Part model, mm, in its own coordinate system. Give positions to 0.01 mm unless a question says otherwise; leave off trailing zeros. Order: outer loops, then holes, each group sorted by start corner. A loop starts at its lowest first (then second) coordinate and runs counter-clockwise, first axis right, second up. Notation, with made-up numbers: (74, -11) - (87, -11) arc R10 cw to (87, -4) - close; hole circle Ø8 at (-17.5, -27). An arc over 180 degrees is marked (long way). One line per item, written item: value.
```python
from build123d import *

# Parameters (mm, degrees)
BOSS_EXTRUDE1_DEPTH     = 28.2702
SKETCH2_R               = 3.556
SKETCH2_R_2             = 1.4986
SKETCH2_R_3             = 2.0066
MOTOR_MOUNT_HOLES_DEPTH = 50.437835996
SKETCH3_R               = 1.7018
PLATE_MOUNT_HOLES_DEPTH = 51.700550556
SKETCH4_W               = 28.2702
SKETCH4_H               = 29.2608
CUT_EXTRUDE1_DEPTH      = 50.437835996
FILLET1_R               = 1.905


with BuildPart() as part:
    # Sketch1 → Boss-Extrude1 (new body)
    with BuildSketch(Plane(origin=(0, 0, 0), x_dir=(0, 0, -1), z_dir=(1, 0, 0))):
        Polygon((0, 0), (0, -30.1498), (-30.2514, -30.1498), (-30.2514, -29.2608), (-3.1242, -29.2608), (-3.1242, 0), align=None)
    extrude(amount=BOSS_EXTRUDE1_DEPTH)

    # Sketch2 → Motor_Mount_holes (cut, through all)
    with BuildSketch(Plane.XY.offset(3.1242)):
        with Locations((14.1351, -11.6586)):
            Circle(SKETCH2_R)
        with Locations((14.1351, -3.1496)):
            Circle(SKETCH2_R_2)
        with Locations((5.2451, -11.6586)):
            Circle(SKETCH2_R_3)
        with Locations(Location((23.0251, -11.6586, 0), (0, 0, 180))):
            Circle(SKETCH2_R_3)
        with Locations(Location((14.1351, -20.1676, 0), (0, 0, 180))):
            Circle(SKETCH2_R_2)
    extrude(amount=-MOTOR_MOUNT_HOLES_DEPTH, mode=Mode.SUBTRACT)

    # Sketch3 → Plate_Mount_Holes (cut, through all)
    with BuildSketch(Plane(origin=(0, -29.2608, 0), x_dir=(1, 0, 0), z_dir=(0, 1, 0))):
        with Locations(Location((24.3205, -7.7597, 0), (0, 0, 270))):
            Circle(SKETCH3_R)
        with Locations(Location((3.9497, -7.7597, 0), (0, 0, 90))):
            Circle(SKETCH3_R)
        with Locations(Location((3.9497, -21.3741, 0), (0, 0, 270))):
            Circle(SKETCH3_R)
        with Locations(Location((24.3205, -21.3741, 0), (0, 0, 90))):
            Circle(SKETCH3_R)
    extrude(amount=-PLATE_MOUNT_HOLES_DEPTH, mode=Mode.SUBTRACT)

    # Sketch4 → Cut-Extrude1 (cut, through all)
    with BuildSketch(Plane.XY.offset(3.1242)):
        with Locations((14.1351, -14.6304)):
            Rectangle(SKETCH4_W, SKETCH4_H)
    extrude(amount=-CUT_EXTRUDE1_DEPTH, mode=Mode.SUBTRACT)

    # Fillet1
    fillet1_edges = [part.edges().sort_by_distance(p)[0] for p in [
        (28.2702, -29.7053, 30.2514),
        (28.2702, -29.7053, 0),
        (0, -29.7053, 0),
        (0, -29.7053, 30.2514),
    ]]
    fillet(fillet1_edges, radius=FILLET1_R)


solid = part.part
```
1) Pin check, flat tip, straight feed: pin 1 (3 mm diameter, centred on x = 3.95, z = 7.76, fed in from -Y). Stop position of the tip, or through.
Outcome:
pin 1: passes through
2) Cut at A-A, the plane x = 25. Give the cut face in (y, z).
Outcome:
outline: (-30.15, 0) - (-29.26, 0) - (-29.26, 6.2) - (-30.15, 6.2) - close; (-30.15, 9.32) - (-29.26, 9.32) - (-29.26, 19.81) - (-30.15, 19.81) - close; (-30.15, 22.93) - (-29.26, 22.93) - (-29.26, 30.25) - (-30.15, 30.25) - close
3) Mould opens along Z. For faces 1 (the cylindrical face through (0.573, -29.712, 0.543)), 2 (the flat face through (14, -30.15, 15)), 3 (the cylindrical face through (4.601, -29.699, 6.188)) say: released by +Z, released by -Z, zero draft, split by the parting line, or undercut.
Outcome:
face 1: released by -Z
face 2: zero draft
face 3: undercut
4) Cut at B-B, the plane z = 9. Give the cut face in (x, y).
Outcome:
outline: (0, -30.15) - (2.78, -30.15) - (2.78, -29.26) - (0, -29.26) - close; (5.11, -30.15) - (23.16, -30.15) - (23.16, -29.26) - (5.11, -29.26) - close; (25.49, -30.15) - (28.27, -30.15) - (28.27, -29.26) - (25.49, -29.26) - close
5) Cut at C-C, the plane y = -29.9. Give the cut face in (x, z) (1 decimal), then the cut area to 3 significant figures.
Outcome:
outline: (0, 1.9) arc R1.9 ccw to (1.9, 0) - (26.4, 0) arc R1.9 ccw to (28.3, 1.9) - (28.3, 28.3) arc R1.9 ccw to (26.4, 30.3) - (1.9, 30.3) arc R1.9 ccw to (0, 28.3) - close; hole circle Ø3.4 at (3.9, 7.8); hole circle Ø3.4 at (3.9, 21.4); hole circle Ø3.4 at (24.3, 7.8); hole circle Ø3.4 at (24.3, 21.4)
area: 816 mm^2
6) Drill centre lines: line 1 along Z through (x, y) = (23.75, -30.1); line 2 along Z through (x, y) = (23, -29.8); line 3 along X through (y, z) = (-29.95, 22.5). Where is each one in solid material? Low to high. Write a range as from..to.
Outcome:
line 1: z = 0..6.16, 9.36..19.77, 22.98..30.25
line 2: z = 0..6.69, 8.83..20.3, 22.45..30.25
line 3: x = 0..2.67, 5.23..23.04, 25.6..28.27
